Autodesk Inventor part; units mm, degrees
ref_plane "YZ Plane" through (0, 0, 0) normal (1, 0, 0) x (0, 1, 0)
ref_plane "XZ Plane" through (0, 0, 0) normal (0, 1, 0) x (-1, 0, 0)
ref_plane "XY Plane" through (0, 0, 0) normal (0, 0, 1) x (1, 0, 0)
sketch "Sketch1" plane through (0, 0, 0) normal (1, 0, 0) x (0, 1, 0)
  line L0 (0, 0) -> (50.8, 0)
  line L1 (0, 138.1125) -> (26.719, 138.1125)
  line L2 (0, 138.1125) -> (0, 169.8625)
  line L3 (0, 169.8625) -> (3.175, 169.8625)
  line L4 (3.175, 169.8625) -> (3.175, 141.2875)
  line L5 (3.175, 141.2875) -> (60.325, 141.2875)
  line L6 (60.325, 141.2875) -> (60.325, 179.3875)
  line L7 (60.325, 179.3875) -> (63.5, 179.3875)
  line L8 (63.5, 179.3875) -> (63.5, 138.1125)
  line L9 (63.5, 138.1125) -> (26.719, 138.1125)
  point P0 (62.1333, 179.3875)
  dimension "d0" = 50.8
  dimension "d1" = 138.1125
  dimension "d2" = 31.75
  dimension "d3" = 3.175
  dimension "d4" = 3.175
  dimension "d5" = 57.15
  dimension "d6" = 38.1
  dimension "d7" = 3.175
revolve "Revolution1" add sketch "Sketch1" angle 360 about axis through (0, 0, 0) along (0, 1, 0)
ref_plane "Work Plane1" through (0, 62.1333, 179.3875) normal (0, 0, 1) x (1, 0, 0)
sketch "Sketch2" plane through (0, 62.1333, 179.3875) normal (0, 0, 1) x (1, 0, 0)
  circle A0 centre (0, -32.8344) radius 6.35
  line L0 (169.8625, -58.9583) -> (-169.8625, -58.9583)
  point P0 (0, -62.1333)
  dimension "d9" = 12.7
  dimension "d10" = 26.1239
extrude "Extrusion1" cut sketch "Sketch2" against normal through all
properties part number "Layer2_Ref"
Verification items for the finished model (mm, model axes). A direction names the side the tool comes from. Give positions to 0.01 mm unless a question says otherwise; leave off trailing zeros. Write each loop counter-clockwise with the first axis right and the second up, starting at its lowest first coordinate (ties: lowest second). Pieces come first, ordered by that corner, then holes. Notation, with made-up numbers: (-7.5, 9) -> (28.5, 9) arc R16 cw to (28.5, 39) -> close; hole circle Ø3 at (26.5, 81). An arc over 180 degrees is marked (long way). Use CSV: the item, a comma, the result in double quotes.
(1) Go/stop test with flat-tipped pins: pin 1 (1 mm diameter, centred on x = -98.5, y = 8, fed in from +Z); pin 2 (16.5 mm diameter, centred on x = 0, y = 29.3, fed in from +Z); pin 3 (1 mm diameter, centred on y = 14, z = 69.5, fed in from -X). Record where each tip stops, or that it passes through.
Derived:
pin 1,"stops at z = 101.78"
pin 2,"stops at z = 141.29"
pin 3,"stops at x = -123.29"
(2) Sectioned sample at D-D (y = 43.5). Record the cut outline in (x, z) (1 decimal).
Derived:
outline,"circle Ø282.6 at (0, 0); hole circle Ø276.2 at (0, 0)"
(3) Sectioned sample at A-A (x = 0). Record the cut outline in (y, z) (1 decimal), plus the area to 3 significant figures.
Derived:
outline,"(0, -169.9) -> (3.2, -169.9) -> (3.2, -141.3) -> (22.9, -141.3) -> (22.9, -138.1) -> (0, -138.1) -> close; (0, 138.1) -> (22.9, 138.1) -> (22.9, 141.3) -> (3.2, 141.3) -> (3.2, 169.9) -> (0, 169.9) -> close; (35.6, -141.3) -> (60.3, -141.3) -> (60.3, -179.4) -> (63.5, -179.4) -> (63.5, -138.1) -> (35.6, -138.1) -> close; (35.6, 138.1) -> (63.5, 138.1) -> (63.5, 179.4) -> (60.3, 179.4) -> (60.3, 141.3) -> (35.6, 141.3) -> close"
area,"746 mm^2"
(4) Sectioned sample at B-B (z = 0). Record the cut outline in (x, y) (1 decimal), plus the area to 3 significant figures.
Derived:
outline,"(-179.4, 60.3) -> (-141.3, 60.3) -> (-141.3, 3.2) -> (-169.9, 3.2) -> (-169.9, 0) -> (-138.1, 0) -> (-138.1, 63.5) -> (-179.4, 63.5) -> close; (138.1, 0) -> (169.9, 0) -> (169.9, 3.2) -> (141.3, 3.2) -> (141.3, 60.3) -> (179.4, 60.3) -> (179.4, 63.5) -> (138.1, 63.5) -> close"
area,"827 mm^2"
(5) Set-up check for faces 1 (the cylindrical face through (-165.823, 1.61, -36.823)), 2 (the flat face through (-132, 60.325, 52)), 3 (the cylindrical face through (53.9, 61.9, 171.1)): record each of +Z, -Z, +X, -X, +Y, -Y from which the full face is reachable in a straight line by a thin tool's end or side.
Derived:
face 1,"-Y"
face 2,"none"
face 3,"+Y, -Y"
(6) Sectioned sample at C-C (x = 52). Record the cut outline in (y, z) (3 decimals).
Derived:
outline,"(0, -161.707) -> (3.175, -161.707) -> (3.175, -131.37) -> (60.325, -131.37) -> (60.325, -171.685) -> (63.5, -171.685) -> (63.5, -127.949) -> (0, -127.949) -> close; (0, 127.949) -> (63.5, 127.949) -> (63.5, 171.685) -> (60.325, 171.685) -> (60.325, 131.37) -> (3.175, 131.37) -> (3.175, 161.707) -> (0, 161.707) -> close"
(7) Material ranges on L1, parallel to Z at x = 0, y = 43; L2, parallel to Y at x = 155, z = -2 (3 decimals), recorded low to high.
Derived:
L1,"z = -141.29 to -138.11, 138.11 to 141.29"
L2,"y = 0 to 3.175, 60.325 to 63.5"
(8) Release check for a two-part mould opening along X. For faces 4 (the cylindrical face through (42.439, 32.15, 134.763)), 5 (the flat face through (139, 0, -1)), 6 (the cylindrical face through (-0.8, 35.6, -139.6)) record: +X half, -X half, draft (parallel to the pull), parting line (faces both ways), or undercut.
Derived:
face 4,"parting line"
face 5,"draft"
face 6,"undercut"
